Input: part model. Units: mm. Frame: model coordinates. A direction names the side the tool comes from. Coordinates: 2 decimals unless noted, no trailing zeros. Write each loop counter-clockwise with the first axis right and the second up, starting at its lowest first coordinate (ties: lowest second). Pieces come first, ordered by that corner, then holes. Notation, with made-up numbers: M -12,31.25 L 14,31.25 A13 cw 14,47.25 Z; hole C -28,-36 d9. An arc over 180 degrees is marked long. Use CSV: the item, a comma, the result in double quotes.
```python
from build123d import *

# Parameters (mm, degrees)
BOSS_EXTRUDE1_DEPTH     = 72
CUT_EXTRUDE2_DEPTH      = 176.28548143
CUT_EXTRUDE2_DEPTH_BACK = 25
SKETCH3_W               = 50
SKETCH3_H               = 6
CUT_EXTRUDE4_DEPTH      = 72
CUT_EXTRUDE6_DEPTH      = 16
SKETCH5_R               = 12
CUT_EXTRUDE7_DEPTH      = 16


with BuildPart() as part:
    # Sketch1 → Boss-Extrude1 (new body)
    with BuildSketch(Plane.XY):
        Polygon((0, 0), (-146, 0), (-146, 90), (-116, 90), (-116, 25), (0, 25), align=None)
    extrude(amount=BOSS_EXTRUDE1_DEPTH)

    # Sketch2 → Cut-Extrude2 (cut, two sides: drawn at the far end of the back side and taken through both)
    with BuildSketch(Plane(origin=(0, 25, 0), x_dir=(1, 0, 0), z_dir=(0, 1, 0)).offset(-CUT_EXTRUDE2_DEPTH_BACK)):
        with BuildLine():
            Line((-50, -48), (0, -48))
            Line((0, -48), (0, -24))
            Line((0, -24), (-50, -24))
            ThreePointArc((-50, -24), (-62, -36), (-50, -48))
        make_face()
    extrude(amount=CUT_EXTRUDE2_DEPTH + CUT_EXTRUDE2_DEPTH_BACK, mode=Mode.SUBTRACT)

    # Sketch3 → Cut-Extrude4 (cut)
    with BuildSketch(Plane.ZY.offset(146)):
        with Locations((47, 3)):
            Rectangle(SKETCH3_W, SKETCH3_H)
    extrude(amount=-CUT_EXTRUDE4_DEPTH, mode=Mode.SUBTRACT)

    # Sketch4 → Cut-Extrude6 (cut)
    with BuildSketch(Plane.ZY.offset(146)):
        with BuildLine():
            Line((12, 66), (0, 66))
            Line((0, 66), (0, 30))
            Line((0, 30), (12, 30))
            ThreePointArc((12, 30), (36, 18), (60, 30))
            Line((60, 30), (72, 30))
            Line((72, 30), (72, 66))
            Line((72, 66), (60, 66))
            ThreePointArc((60, 66), (36, 78), (12, 66))
        make_face()
    extrude(amount=-CUT_EXTRUDE6_DEPTH, mode=Mode.SUBTRACT)

    # Sketch5 → Cut-Extrude7 (cut)
    with BuildSketch(Plane.ZY.offset(130)):
        with Locations((36, 48)):
            Circle(SKETCH5_R)
    extrude(amount=-CUT_EXTRUDE7_DEPTH, mode=Mode.SUBTRACT)


solid = part.part
```
1. Section B-B (z = 36). Return loops of the section in (x, y).
Resolved:
outline,"M -146,6 L -74,6 L -74,0 L -62,0 L -62,25 L -116,25 L -116,36 L -130,36 L -130,18 L -146,18 Z; M -146,78 L -130,78 L -130,60 L -116,60 L -116,90 L -146,90 Z"
2. Material intervals for line 1 (Y direction, x = -121.5, z = 36); line 2 (Y direction, x = -95.5, z = 10); line 3 (X direction, y = 38, z = 49), sorted ascending. Write a range as [from, to].
Resolved:
line 1,"y = [6, 36], [60, 90]"
line 2,"y = [0, 25]"
line 3,"x = [-130, -116]"
3. Access query for faces 4 (the cylindrical face through (-138, 78, 36)), 5 (the flat face through (-138, 30, 66)), 6 (the flat face through (-25, 12, 48)), 7 (the flat face through (-116, 65, 35)). Directions: +Z, -Z, +X, -X, +Y, -Y. A direction counts if a zero-diameter tool reaches every point of the face in a straight line with its end or side. Return the directions, or none.
Resolved:
face 4,"-X"
face 5,"+Z, -Z, -X"
face 6,"+X, +Y, -Y"
face 7,"+Z, -Z, +X, +Y"
4. Section C-C (x = -14.5). Return loops of the section in (y, z), then the cut area to 3 significant figures.
Resolved:
outline,"M 0,0 L 25,0 L 25,24 L 0,24 Z; M 0,48 L 25,48 L 25,72 L 0,72 Z"
area,"1,200 mm^2"
5. Mould query, pull axis Z, two halves, no side actions, for faces 1 (the flat face through (-131, 90, 35)), 2 (the flat face through (-25, 12, 24)), 3 (the flat face through (-111, 3, 22)). Classes: pulls with the +Z half, pulls with the -Z half, needs draft (parallel to the pull), parting line crosses it, or undercut.
Resolved:
face 1,"needs draft"
face 2,"undercut"
face 3,"pulls with the +Z half"
6. Section A-A (y = 48). Return loops of the section in (x, z).
Resolved:
outline,"M -130,0 L -116,0 L -116,24 L -130,24 Z; M -130,48 L -116,48 L -116,72 L -130,72 Z"
7. Section D-D (z = 63). Return loops of the section in (x, y).
Resolved:
outline,"M -146,6 L -74,6 L -74,0 L 0,0 L 0,25 L -116,25 L -116,90 L -146,90 L -146,66 L -130,66 L -130,30 L -146,30 Z"
8. Contact query for flat-ended pins moving along their axis: pin 1 Ø3 at (x, z) = (-72, 59.5) entering from -Y; pin 2 Ø15 at (x, z) = (-116, 38) entering from -Y; pin 3 Ø18 at (y, z) = (56.5, 53) entering from -X; pin 4 Ø19.5 at (y, z) = (61, 33.5) entering from +X. Output: stop coordinate, or through.
Resolved:
pin 1,"stops at y = 0"
pin 2,"stops at y = 6"
pin 3,"stops at x = -130"
pin 4,"stops at x = -116"
